Here's the drawing with two shaded views (mm, measured from the low corner). I have some questions. A direction names the side the tool comes from. Coordinates: 2 decimals unless noted, no trailing zeros. Loops run counter-clockwise (first coordinate to the right, second up) from the corner with the lowest first, then second, coordinate; pieces in that order, holes last. Notation, with made-up numbers: (15, 9) - (43, 9) arc R25 ccw to (43, 42) - close; hole circle Ø10 at (-4, -23.75). An arc over 180 degrees is marked (long way). Use a Markdown table: item, result.
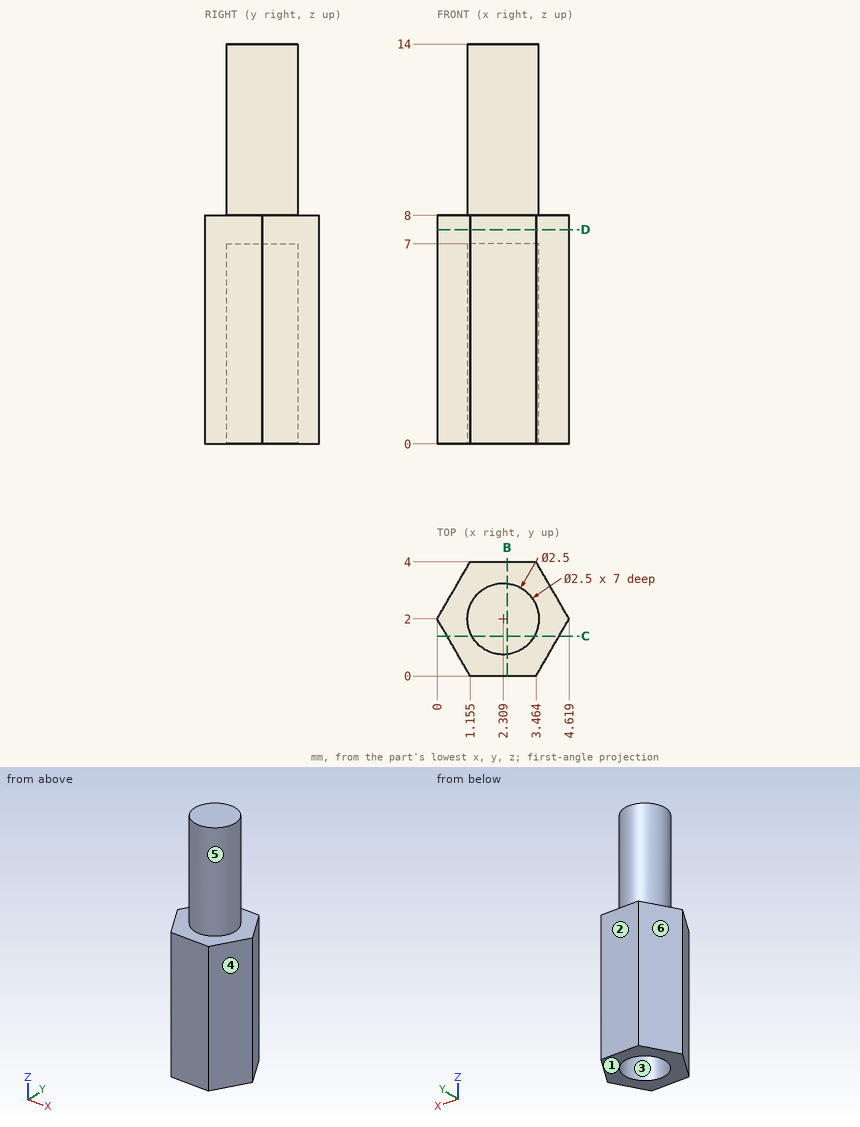
Q1. Please list where these lines run through material, in increasing order: L1, parallel to Z at x = 1, y = 2.35; L2, parallel to Z at x = 3, y = 2.2; L3, parallel to Y at x = 3.05, z = 6.5 (1 decimal). Write a range as from..to.
Check values:
| item | result |
|---|---|
| L1 | 0..8 |
| L2 | 7..14 |
| L3 | 0..1, 3..4 |
Q2. I want a section at B-B, the plane x = 2.45. Write out the boundary of the cut face in (y, z).
Check values:
| item | result |
|---|---|
| outline | (0, 0) - (0.76, 0) - (0.76, 7) - (3.24, 7) - (3.24, 0) - (4, 0) - (4, 8) - (3.24, 8) - (3.24, 14) - (0.76, 14) - (0.76, 8) - (0, 8) - close |
Q3. I want a section at C-C, the plane y = 1.4. Write out the boundary of the cut face in (x, z).
Check values:
| item | result |
|---|---|
| outline | (0.35, 0) - (1.21, 0) - (1.21, 7) - (3.41, 7) - (3.41, 0) - (4.27, 0) - (4.27, 8) - (3.41, 8) - (3.41, 14) - (1.21, 14) - (1.21, 8) - (0.35, 8) - close |
Q4. Which directions (+Z, -Z, +X, -X, +Y, -Y) give clear straight access to the entire face, cutting with the end or side of a thin tool? Please do the marked faces 5 and 6.
Check values:
| item | result |
|---|---|
| face 5 | +Z |
| face 6 | +Z, -Z, -X, +Y |
Q5. Will these pins go through, and if not, where does the flat tip stop? P1, Ø1.2, axis at x = 2.5, y = 2, coming from the -Z side; P2, Ø2, axis at y = 3.5, z = 12, coming from the +X side (1 decimal); P3, Ø1.5, axis at y = 3, z = 4, coming from the +X side (1 decimal).
Check values:
| item | result |
|---|---|
| P1 | z = 7 |
| P2 | x = 3.5 |
| P3 | x = 4.5 |
Q6. If we mould it in two halves opening along Y, with no side actions, what happens to the marked faces 1, 2, 3 and 4? For each: pulls with the +Y half, pulls with the -Y half, needs draft (parallel to the pull), parting line crosses it, or undercut.
Check values:
| item | result |
|---|---|
| face 1 | needs draft |
| face 2 | pulls with the +Y half |
| face 3 | undercut |
| face 4 | pulls with the -Y half |
Q7. I want a section at D-D, the plane z = 7.5. Write out the boundary of the cut face in (x, y) (1 decimal).
Check values:
| item | result |
|---|---|
| outline | (0, 2) - (1.2, 0) - (3.5, 0) - (4.6, 2) - (3.5, 4) - (1.2, 4) - close |
